```python
from build123d import *

# Parameters (mm, degrees)
SZKIC1_R                    = 12
DODANIE_WYCI_GNI_CIE1_DEPTH = 15
SZKIC6_R                    = 3.25
WYTNIJ_WYCI_GNI_CIE5_DEPTH  = 16
SZKIC8_W                    = 15
SZKIC8_H                    = 50
WYTNIJ_WYCI_GNI_CIE6_DEPTH  = 7.5
SZKIC9_R                    = 2.5
WYTNIJ_WYCI_GNI_CIE7_DEPTH  = 10
SZYK_KO_OWY1_COUNT          = 4
SFAZOWANIE1_SIZE            = 0.5
SZKIC10_R                   = 35
WYTNIJ_WYCI_GNI_CIE8_DEPTH  = 3


with BuildPart() as part:
    # Szkic1 → Dodanie-wyci_gni_cie1 (new body)
    with BuildSketch(Plane.XY):
        Polygon((42.5, 25), (42.5, 42.5), (-42.5, 42.5), (-42.5, 25), (-57.5, 25), (-57.5, -25), (-42.5, -25), (-42.5, -42.5), (42.5, -42.5), (42.5, -25), (57.5, -25), (57.5, 25), align=None)
        Circle(SZKIC1_R, mode=Mode.SUBTRACT)
    extrude(amount=DODANIE_WYCI_GNI_CIE1_DEPTH)

    # Szkic6 → Wytnij-wyci_gni_cie5 (cut, through all)
    with BuildSketch(Plane(origin=(0, 0, 0), x_dir=(-1, 0, 0), z_dir=(0, 0, -1))):
        with Locations((-50, -15)):
            Circle(SZKIC6_R)
        with Locations((-50, 15)):
            Circle(SZKIC6_R)
        with Locations((50, 15)):
            Circle(SZKIC6_R)
        with Locations((50, -15)):
            Circle(SZKIC6_R)
    extrude(amount=-WYTNIJ_WYCI_GNI_CIE5_DEPTH, mode=Mode.SUBTRACT)

    # Szkic8 → Wytnij-wyci_gni_cie6 (cut)
    with BuildSketch(Plane.XY.offset(15)):
        with Locations((-50, 0)):
            Rectangle(SZKIC8_W, SZKIC8_H)
        with Locations((50, 0)):
            Rectangle(SZKIC8_W, SZKIC8_H)
    extrude(amount=-WYTNIJ_WYCI_GNI_CIE6_DEPTH, mode=Mode.SUBTRACT)

    # Szkic9 → Wytnij-wyci_gni_cie7 (cut)
    with BuildSketch(Plane(origin=(0, 0, 0), x_dir=(-1, 0, 0), z_dir=(0, 0, -1))):
        with Locations((-31.819805153, 31.819805153)):
            Circle(SZKIC9_R)
    wytnij_wyci_gni_cie7 = extrude(amount=-WYTNIJ_WYCI_GNI_CIE7_DEPTH, mode=Mode.SUBTRACT)

    # Szyk ko_owy1: Wytnij-wyci_gni_cie7 ×4 about axis
    szyk_ko_owy1_axis = Axis((0, 0, 0), (0, 0, 1))
    for i in range(1, SZYK_KO_OWY1_COUNT):
        add(wytnij_wyci_gni_cie7.rotate(szyk_ko_owy1_axis, i * 360 / SZYK_KO_OWY1_COUNT), mode=Mode.SUBTRACT)

    # Sfazowanie1
    sfazowanie1_edges = [part.edges().sort_by_distance(p)[0] for p in [
        (31.819805153, -34.319805153, 0),
        (-34.319805153, -31.819805153, 0),
        (-31.819805153, 34.319805153, 0),
        (34.319805153, 31.819805153, 0),
    ]]
    chamfer(sfazowanie1_edges, length=SFAZOWANIE1_SIZE)

    # Szkic10 → Wytnij-wyci_gni_cie8 (cut)
    with BuildSketch(Plane(origin=(0, 0, 0), x_dir=(-1, 0, 0), z_dir=(0, 0, -1))):
        Circle(SZKIC10_R)
    extrude(amount=-WYTNIJ_WYCI_GNI_CIE8_DEPTH, mode=Mode.SUBTRACT)


solid = part.part
```
Work out the finished part from the listing and answer in its coordinate system (mm). A direction names the side the tool comes from. Coordinates: 2 decimals unless noted, no trailing zeros. Order: outer loops, then holes, each group sorted by start corner. A loop starts at its lowest first (then second) coordinate and runs counter-clockwise, first axis right, second up. Notation, with made-up numbers: M -3.5,20 L 47.5,20 A23 ccw 47.5,38 Z; hole C -19.5,46.5 d10. An arc over 180 degrees is marked long. Use CSV: the item, a comma, the result in double quotes.
1) Section D-D on z = 5.5 is taken. Count the separate pieces of the cut face and the enclosed holes in it, plus the area to 3 significant figures.
Worked out:
separate pieces,"1"
enclosed holes,"9"
area,"8,060 mm^2"
2) Section C-C on x = 0 is taken. Write down the section's boundary in (y, z), plus the area to 3 significant figures.
Worked out:
outline,"M -42.5,0 L -35,0 L -35,3 L -12,3 L -12,15 L -42.5,15 Z; M 12,3 L 35,3 L 35,0 L 42.5,0 L 42.5,15 L 12,15 Z"
area,"777 mm^2"
3) Determine the mould class of faces 5 (the face through (-1, -42.5, 7)), 6 (the face through (-32, -32, 10)) for opening direction X: released by +X, released by -X, zero draft, split by the parting line, or undercut.
Worked out:
face 5,"zero draft"
face 6,"undercut"
4) Section B-B on y = 0 is taken. Write down the section's boundary in (x, z).
Worked out:
outline,"M -57.5,0 L -35,0 L -35,3 L -12,3 L -12,15 L -42.5,15 L -42.5,7.5 L -57.5,7.5 Z; M 12,3 L 35,3 L 35,0 L 57.5,0 L 57.5,7.5 L 42.5,7.5 L 42.5,15 L 12,15 Z"
5) Consider line 1 (Y direction, x = -50, z = 5.25); line 2 (X direction, y = 14, z = 1); line 3 (Y direction, x = -51.5, z = 6.25). Determine where each line is inside the solid, lowest interval first. Write a range as [from, to].
Worked out:
line 1,"y = [-25, -18.25], [-11.75, 11.75], [18.25, 25]"
line 2,"x = [-57.5, -53.09], [-46.91, -32.08], [32.08, 46.91], [53.09, 57.5]"
line 3,"y = [-25, -17.88], [-12.12, 12.12], [17.88, 25]"
6) Flat-ended cylindrical pins translate along their axes: pin 1 Ø8 at (y, z) = (-30, 12) entering from +X; pin 2 Ø6 at (x, z) = (-48.5, 3.5) entering from -Y; pin 3 Ø6 at (x, z) = (48.5, 4.5) entering from +Y. Find the tip coordinate at first contact, or state that the pin passes through.
Worked out:
pin 1,"stops at x = 42.5"
pin 2,"stops at y = -25"
pin 3,"stops at y = 25"
7) Section A-A on x = 50 is taken. Write down the section's boundary in (y, z).
Worked out:
outline,"M -25,0 L -18.25,0 L -18.25,7.5 L -25,7.5 Z; M -11.75,0 L 11.75,0 L 11.75,7.5 L -11.75,7.5 Z; M 18.25,0 L 25,0 L 25,7.5 L 18.25,7.5 Z"
8) For faces 1 (the face through (50, 0, 7.5)), 2 (the face through (50, 25, 4)), 3 (the face through (-50, 0, 7.5)), 4 (the face through (29.6, -30.67, 5.18)), determine the directions among +Z, -Z, +X, -X, +Y, -Y from which every point of the face is accessible in a straight line to the end or side of a thin tool.
Worked out:
face 1,"+Z, +X, +Y, -Y"
face 2,"+Z, -Z, +X, +Y"
face 3,"+Z, -X, +Y, -Y"
face 4,"-Z"
